Geometry check sheet. Reference: the model listing, model coordinates, mm. Face numbers are marked on the shaded views. Coordinates: 2 decimals unless noted, no trailing zeros. Loops run counter-clockwise (first coordinate to the right, second up) from the corner with the lowest first, then second, coordinate; pieces in that order, holes last. Notation, with made-up numbers: (48.5, 73) -> (98.5, 73) arc R10 ccw to (98.5, 82) -> close; hole circle Ø2 at (-32, 84.25). An arc over 180 degrees is marked (long way). Answer as a JSON object with one key per item and string values.
from build123d import *

# Parameters (mm, degrees)
F0_R     = 9.525
F1_DEPTH = 19.05


with BuildPart() as f1:
    # F0 (on Front) → F1 (new body)
    with BuildSketch(Plane.XZ):
        with BuildLine():
            ThreePointArc((-79.629, 56.773823), (-109.026427, 58.618396), (-110.871, 29.220969))
            ThreePointArc((-110.871, 29.220969), (0, -20.828), (110.871, 29.220969))
            ThreePointArc((110.871, 29.220969), (109.026427, 58.618396), (79.629, 56.773823))
            ThreePointArc((79.629, 56.773823), (0, 20.828), (-79.629, 56.773823))
        make_face()
        with Locations((-95.25, 42.997396)):
            Circle(F0_R, mode=Mode.SUBTRACT)
        with Locations((95.25, 42.997396)):
            Circle(F0_R, mode=Mode.SUBTRACT)
    extrude(amount=F1_DEPTH)


solid = f1.part
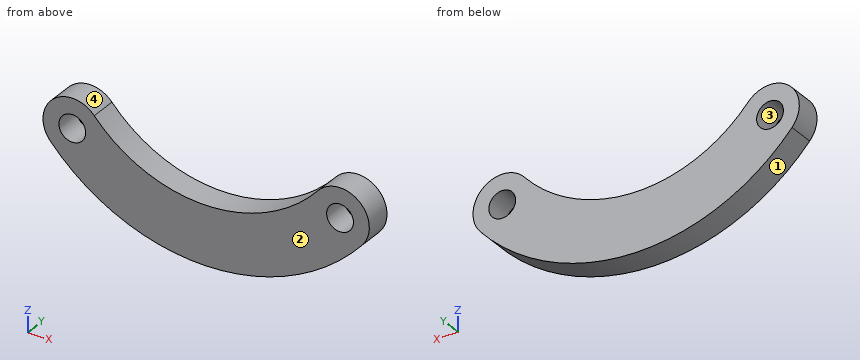
1. Thickness scan on probe 1 along X at (y, z) = (-12.25, 41); probe 2 along Z at (x, y) = (95.25, -12); probe 3 along Z at (x, y) = (-101, -0.75). Record the ranges inside material, lowest first. Write a range as from..to.
Evaluation:
{"probe 1": "x = -115.98..-104.56, -85.94..-62.26, 62.26..85.94, 104.56..115.98", "probe 2": "z = 13.95..33.47, 52.52..63.83", "probe 3": "z = 19.06..35.4, 50.59..63.02"}
2. Section check A-A, the plane z = 47.5. Record the boundary of the cut face in (x, y).
Evaluation:
{"outline": "(-115.59, -19.05) -> (-103.64, -19.05) -> (-103.64, 0) -> (-115.59, 0) -> close; (-86.86, -19.05) -> (-70.37, -19.05) -> (-70.37, 0) -> (-86.86, 0) -> close; (70.37, -19.05) -> (86.86, -19.05) -> (86.86, 0) -> (70.37, 0) -> close; (103.64, -19.05) -> (115.59, -19.05) -> (115.59, 0) -> (103.64, 0) -> close"}
3. Section check B-B, the plane x = 95.25. Record the boundary of the cut face in (y, z).
Evaluation:
{"outline": "(-19.05, 13.95) -> (0, 13.95) -> (0, 33.47) -> (-19.05, 33.47) -> close; (-19.05, 52.52) -> (0, 52.52) -> (0, 63.83) -> (-19.05, 63.83) -> close"}
4. Section check C-C, the plane y = -6.25. Record the boundary of the cut face in (x, z) (3 decimals).
Evaluation:
{"outline": "(-110.871, 29.221) arc R147.828 ccw to (110.871, 29.221) arc R20.828 ccw to (79.629, 56.774) arc R106.172 cw to (-79.629, 56.774) arc R20.828 ccw to start; hole circle Ø19.05 at (-95.25, 42.997); hole circle Ø19.05 at (95.25, 42.997)"}
5. Section check D-D, the plane x = -29. Record the boundary of the cut face in (y, z).
Evaluation:
{"outline": "(-19.05, -17.96) -> (0, -17.96) -> (0, 24.87) -> (-19.05, 24.87) -> close"}
6. Mould release check, pull along Z, two halves, no side actions. Record for the marked faces 1, 2, 3 and 4: released by +Z, released by -Z, zero draft, split by the parting line, or undercut.
Evaluation:
{"face 1": "released by -Z", "face 2": "zero draft", "face 3": "undercut", "face 4": "split by the parting line"}
7. Depth check by flat-ended pin: P1, Ø15, axis at x = -95.25, z = 43, coming from the +Y side; P2, Ø5, axis at y = -8, z = -12.5, coming from the +X side; P3, Ø6, axis at x = 75.5, y = -4.5, coming from the +Z side; P4, Ø5, axis at x = -70.5, y = -8, coming from the +Z side. Enter the tip coordinate at first touch or a pass-through.
Evaluation:
{"P1": "passes through", "P2": "stops at x = 55.53", "P3": "stops at z = 55.51", "P4": "stops at z = 49.91"}
